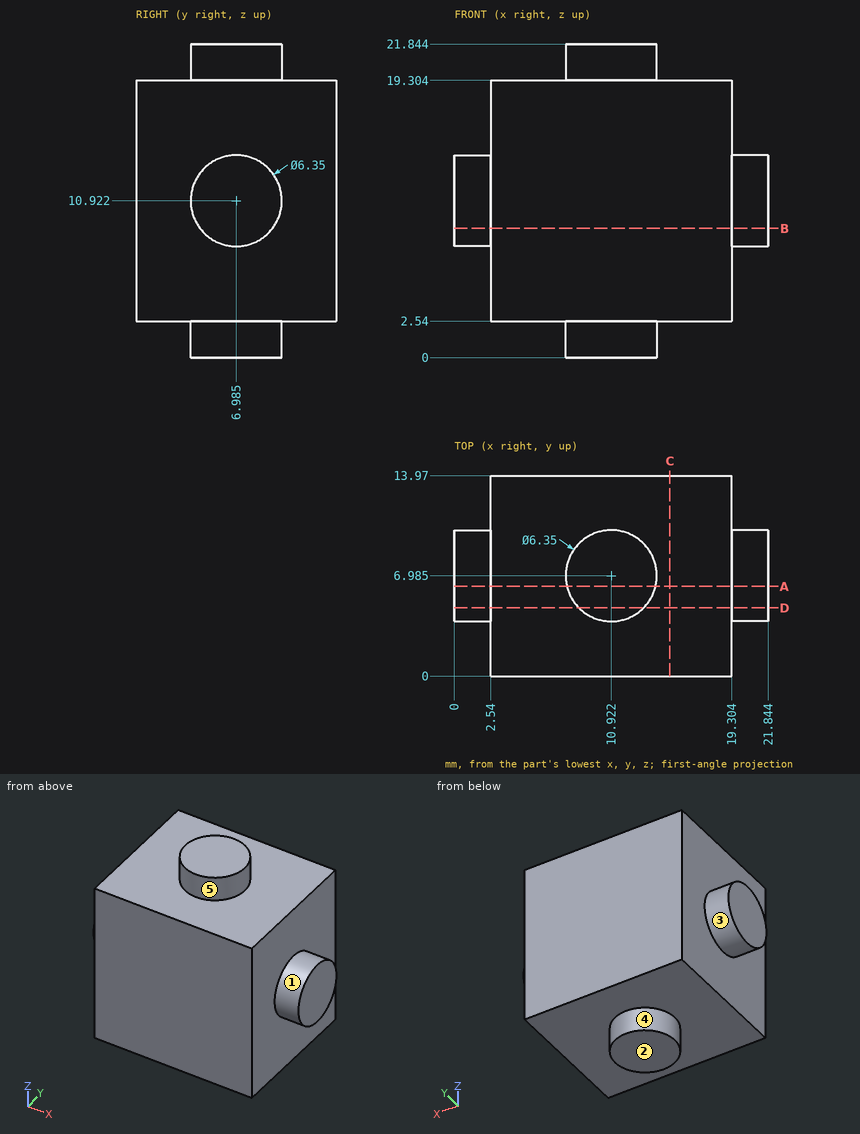
Geometry check sheet. Reference: drawing and pictorial views, mm from the part's lowest x, y, z. A direction names the side the tool comes from. Round coordinates to 2 decimals unless told otherwise and drop trailing zeros. Write each loop counter-clockwise with the first axis right and the second up, starting at its lowest first coordinate (ties: lowest second). Pieces come first, ordered by that corner, then holes.
1. Scan lines: L1, parallel to X at y = 7, z = 19; L2, parallel to Y at x = 19.75, z = 9.5. Record each from-to range of solid material in increasing order.
2. Access from +Z, -Z, +X, -X, +Y, -Y to the whole of each face (thin tool, end or side, straight path). Record for the marked faces 1, 2, 3, 4 and 5.
3. Section check C-C on x = 15. Enter the section's corners in (y, z).
4. Section check A-A on y = 6.25. Enter the section's corners in (x, z).
5. Section check B-B on z = 9. Enter the section's corners in (x, y), plus the area to 3 significant figures.
6. Section check D-D on y = 4.75. Enter the section's corners in (x, z).
7. Gauge pin test, flat ends, axial feed: P1, Ø2, axis at x = 15, y = 10.5, coming from the -Z side; P2, Ø4, axis at x = 3, z = 17.5, coming from the -Y side; P3, Ø2, axis at y = 1.5, z = 5.5, coming from the -X side. Record the tip position at first contact, or that the pin passes through.
Answer:
1. L1: x = 2.54 to 19.3
1. L2: y = 4.15 to 9.82
2. face 1: +X
2. face 2: -Z, +X, -X, +Y, -Y
2. face 3: -X
2. face 4: -Z
2. face 5: +Z
3. outline: (0, 2.54) - (13.97, 2.54) - (13.97, 19.3) - (0, 19.3) - close
4. outline: (0, 7.83) - (2.54, 7.83) - (2.54, 2.54) - (7.83, 2.54) - (7.83, 0) - (14.01, 0) - (14.01, 2.54) - (19.3, 2.54) - (19.3, 7.83) - (21.84, 7.83) - (21.84, 14.01) - (19.3, 14.01) - (19.3, 19.3) - (14.01, 19.3) - (14.01, 21.84) - (7.83, 21.84) - (7.83, 19.3) - (2.54, 19.3) - (2.54, 14.01) - (0, 14.01) - close
5. outline: (0, 4.46) - (2.54, 4.46) - (2.54, 0) - (19.3, 0) - (19.3, 4.46) - (21.84, 4.46) - (21.84, 9.51) - (19.3, 9.51) - (19.3, 13.97) - (2.54, 13.97) - (2.54, 9.51) - (0, 9.51) - close
5. area: 260 mm2
6. outline: (0, 8.67) - (2.54, 8.67) - (2.54, 2.54) - (8.67, 2.54) - (8.67, 0) - (13.18, 0) - (13.18, 2.54) - (19.3, 2.54) - (19.3, 8.67) - (21.84, 8.67) - (21.84, 13.18) - (19.3, 13.18) - (19.3, 19.3) - (13.18, 19.3) - (13.18, 21.84) - (8.67, 21.84) - (8.67, 19.3) - (2.54, 19.3) - (2.54, 13.18) - (0, 13.18) - close
7. P1: stops at z = 2.54
7. P2: stops at y = 0
7. P3: stops at x = 2.54
